Model file for the job. Use its own axes, mm. A direction names the side the tool comes from. Round coordinates to 2 decimals unless told otherwise and drop trailing zeros. Order: outer loops, then holes, each group sorted by start corner. A loop starts at its lowest first (then second) coordinate and runs counter-clockwise, first axis right, second up. Notation, with made-up numbers: (82.5, 8) - (111.5, 8) arc R25 cw to (111.5, 24) - close; hole circle Ø4 at (38, -15). An arc over 180 degrees is marked (long way). Answer as CSV lines item,"result". Start each with the question number.
1. Band-saw the part on A-A on x = 10.5. List the corners of the cut face in (y, z).
2. Wall check: line 1 along X through (y, z) = (-0.75, 0); line 2 along X through (y, z) = (-1.25, -1.1); line 3 along Z through (x, y) = (6.75, -0.5). Give the ranges that are in metal, low to high. Write a range as [from, to].
3. 3-axis set-ups, long thin cutter, end or side, ignore diameter. For faces 4 (the face through (-0.8, 0, -1)), 5 (the face through (0, 0, -0.75)), 6 (the face through (8.65, -1.5, 0.07)): which of +Z, -Z, +X, -X, +Y, -Y reach the whole face in a straight line?
4. Pull direction Y, two halves, no side cores. Call faces 1 (the face through (16, 0, 0)), 2 (the face through (0.51, -1.07, -0.82)), 3 (the face through (1.558, -0.127, -0.028)): released by +Y, released by -Y, zero draft, split by the parting line, or undercut.
5. Pin check, flat tips, straight feed: pin 1 Ø3 at (x, z) = (9.5, 0) entering from +Y; pin 2 Ø1 at (x, y) = (3, 0.5) entering from -Z; pin 3 Ø2 at (x, y) = (4.5, -0.5) entering from +Z. Stop position of each tip, or through.
Autodesk Inventor part; units mm, degrees
ref_plane "YZ Plane" through (0, 0, 0) normal (1, 0, 0) x (0, 1, 0)
ref_plane "XZ Plane" through (0, 0, 0) normal (0, 1, 0) x (-1, 0, 0)
ref_plane "XY Plane" through (0, 0, 0) normal (0, 0, 1) x (1, 0, 0)
sketch "Sketch_1" plane through (0, 0, 0) normal (0, 0, 1) x (1, 0, 0)
  line L0 (16, 0) -> (-0.8, 0)
  line L1 (-0.8, 0) -> (-0.8, 2)
  line L2 (-0.8, 2) -> (-0.2226, 3)
  line L3 (-0.2226, 3) -> (0, 3)
  line L4 (0, 3) -> (0, 1.4467)
  arc A0 (0, 1.4467) -> (0.1, 1.3467) centre (0.1, 1.4467) ccw
  line L5 (0.1, 1.3467) -> (0.9, 1.3467)
  line L6 (0.9, 1.3467) -> (1.4, 1.5)
  line L7 (1.4, 1.5) -> (15.6935, 1.5)
  line L8 (15.6935, 1.5) -> (16, 1.1935)
  line L9 (16, 1.1935) -> (16, 0)
  line L10 (16, 0) -> (-0.8, 0)
revolve "Revolution1" add sketch "Sketch_1" angle 360 about axis through (16, 0, 0) along (1, 0, 0)
thread "Thread1"
sketch "Sketch2" plane through (-0.8, 0, 0) normal (-1, 0, 0) x (0, 0, 1)
  point P0 (0, 0)
hole "Hole1" at (-0.8, 0, 0) direction (1, 0, 0) diameter 1.5 depth 2 tip angle 120
sketch "Sketch_3" plane through (-0.8, 0, 0) normal (1, 0, 0) x (0, 0, -1)
  line L0 (-0.75, -0.433) -> (0, -0.866)
  line L1 (0, -0.866) -> (0.75, -0.433)
  line L2 (0.75, -0.433) -> (0.75, 0.433)
  line L3 (0.75, 0.433) -> (0, 0.866)
  line L4 (0, 0.866) -> (-0.75, 0.433)
  line L5 (-0.75, 0.433) -> (-0.75, -0.433)
extrude "Extrusion1" cut sketch "Sketch_3" along normal blind 2
properties part number "CBSTNR3-16" material "鋼、炭素鋼"
Reply:
1,outline,"circle Ø3 at (0, 0)"
2,line 1,"x = [1.2, 16]"
2,line 2,"x = [-0.8, 0]"
2,line 3,"z = [-1.41, 1.41]"
3,face 4,"+Z, -Z, -X, +Y, -Y"
3,face 5,"-X"
3,face 6,"+X"
4,face 1,"zero draft"
4,face 2,"split by the parting line"
4,face 3,"undercut"
5,pin 1,"stops at y = 1.5"
5,pin 2,"stops at z = -1.5"
5,pin 3,"stops at z = 1.5"
